Study the drawing (mm; zero at the part's minimum x, y, z) and answer. Coordinates: 2 decimals unless noted, no trailing zeros. Write each loop counter-clockwise with the first axis right and the second up, starting at its lowest first coordinate (ties: lowest second). Pieces come first, ordered by that corner, then holes. Notation, with made-up numbers: (66.25, 30) - (124.25, 30) arc R17 ccw to (124.25, 60) - close; hole circle Ø9 at (7.5, 7). An arc over 180 degrees is marked (long way). One line per item, written item: value.
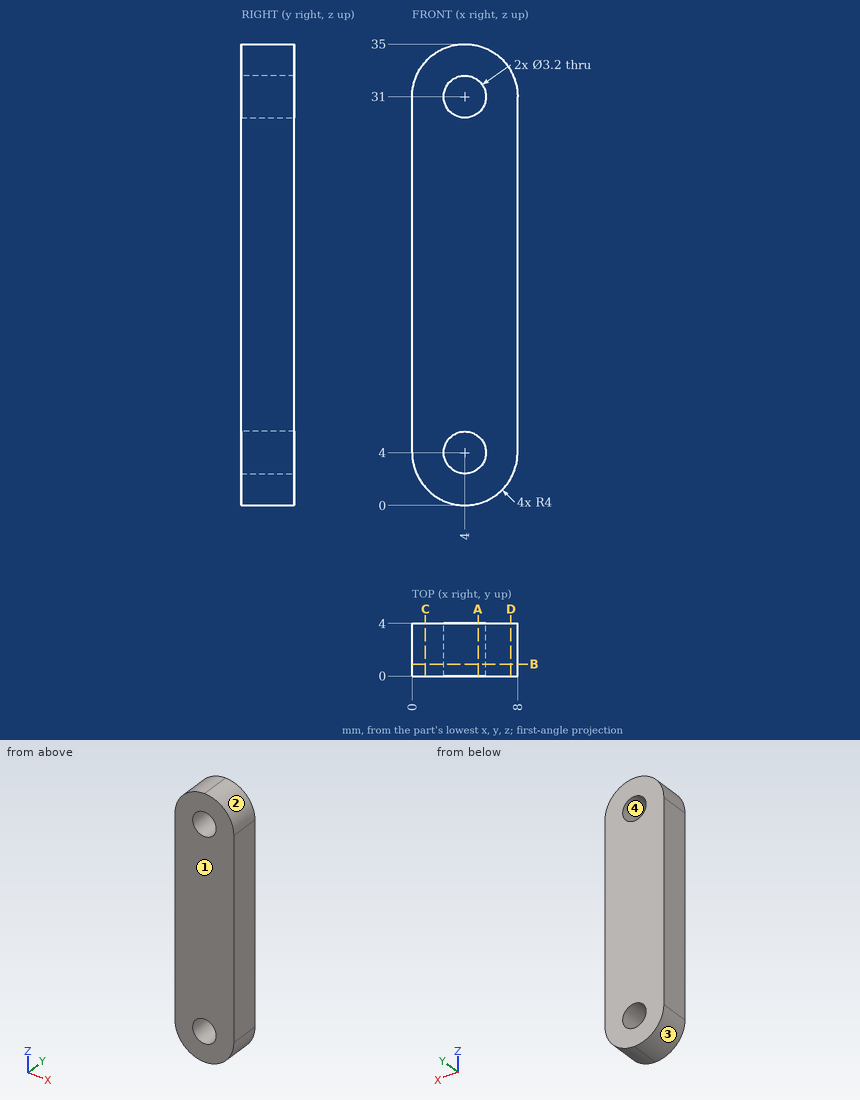
Item 1: Given pin 1 (2 mm diameter, centred on y = 1, z = 28.5, fed in from -X); pin 2 (2.5 mm diameter, centred on x = 4, z = 4, fed in from +Y); pin 3 (1.5 mm diameter, centred on x = 2, y = 3, fed in from +Z); pin 4 (1 mm diameter, centred on x = 5, y = 1, fed in from -Z), each flat-ended and moving along its own axis, determine where each tip first touches the part or whether it passes through.
Evaluation:
pin 1: stops at x = 0
pin 2: passes through
pin 3: stops at z = 34.8
pin 4: stops at z = 0.03
Item 2: Section A-A, the plane x = 5 is taken. Determine the outline of the cut face in (y, z), then the cut area to 3 significant figures.
Evaluation:
outline: (0, 0.13) - (4, 0.13) - (4, 2.75) - (0, 2.75) - close; (0, 5.25) - (4, 5.25) - (4, 29.75) - (0, 29.75) - close; (0, 32.25) - (4, 32.25) - (4, 34.87) - (0, 34.87) - close
area: 119 mm2
Item 3: Determine the mould class of the marked faces 1, 2, 3 and 4 for opening direction Z: +Z half, -Z half, draft (parallel to the pull), parting line (faces both ways), or undercut.
Evaluation:
face 1: draft
face 2: +Z half
face 3: -Z half
face 4: undercut
Item 4: Consider probe 1 along X at (y, z) = (1.4, 4); probe 2 along Z at (x, y) = (4.5, 0.7); probe 3 along Z at (x, y) = (3, 0.95). Determine where each line is inside the solid, lowest interval first.
Evaluation:
probe 1: x = 0 to 2.4, 5.6 to 8
probe 2: z = 0.03 to 2.48, 5.52 to 29.48, 32.52 to 34.97
probe 3: z = 0.13 to 2.75, 5.25 to 29.75, 32.25 to 34.87
Item 5: Section D-D, the plane x = 7.5 is taken. Determine the outline of the cut face in (y, z), then the cut area to 4 significant figures.
Evaluation:
outline: (0, 2.06) - (4, 2.06) - (4, 32.94) - (0, 32.94) - close
area: 123.5 mm2
Item 6: Section B-B, the plane y = 0.9 is taken. Give the number of separate pieces and of enclosed holes in the cut face, then the cut area to 3 significant figures.
Evaluation:
separate pieces: 1
enclosed holes: 2
area: 250 mm2
Item 7: Section C-C, the plane x = 1 is taken. Determine the outline of the cut face in (y, z), then the cut area to 3 significant figures.
Evaluation:
outline: (0, 1.35) - (4, 1.35) - (4, 33.65) - (0, 33.65) - close
area: 129 mm2
